For this review, take the finished solid that the model builds, in its own axes (mm). Face numbers are marked on the shaded views. A direction names the side the tool comes from. Coordinates: 2 decimals unless noted, no trailing zeros. Loops run counter-clockwise (first coordinate to the right, second up) from the corner with the lowest first, then second, coordinate; pieces in that order, holes last. Notation, with made-up numbers: (-38, 11) - (4, 11) arc R25 ccw to (4, 47) - close; hole circle Ø8 at (7, 44.5). An arc over 180 degrees is marked (long way). One line per item, written item: value. Start each with the question number.
1. To check wall thickness, follow line 1 (Z direction, x = 44.25, y = -91); line 2 (Z direction, x = 44, y = 46.5); line 3 (Z direction, x = 45.5, y = 78). State the ranges of each line that lie inside material, in increasing order. Write a range as from..to.
2. For the marked faces 1, 2 and 3, list the 3-axis set-ups (+Z, -Z, +X, -X, +Y, -Y) from which the entire face can be reached by the end or side of a thin tool; tool diameter is ignored.
3. The part is to be moulded in two halves that separate along Y. For the marked faces 4, 5 and 6, say which applies: released by +Y, released by -Y, zero draft, split by the parting line, or undercut.
4. Take a section at B-B, the plane z = -11. State the section outline as (x, y) points.
5. Take a section at C-C, the plane y = -70. State the section outline as (x, z) points, and give its area (3 significant figures).
6. Take a section at D-D, the plane x = 68. State the section outline as (y, z) points, and give its area (3 significant figures).
7. Insertion check: pin 1 (25 mm diameter, centred on x = 58.5, y = -33.5, fed in from +Z); pin 2 (1.8 mm diameter, centred on y = 0, z = 89.5, fed in from -X). Each pin has a flat end and moves straight along its axis. Give the tip position at first contact, or say it passes through.
8. Take a section at A-A, the plane x = 9.25. State the section outline as (y, z) points, and give its area (3 significant figures).
```python
from build123d import *

# Parameters (mm, degrees)
F1_DEPTH = 88.5
F2_R     = 3.4
F3_DEPTH = 30
F5_DEPTH = 208


with BuildPart() as f1:
    # F0 (on Right) → F1 (new body)
    with BuildSketch(Plane.YZ):
        Polygon((-74.5, 0), (68.5, 0), (56.952995, -20), (103.5, -20), (103.5, 85), (-104.5, 85), (-104.5, -20), (-74.5, -20), align=None)
    extrude(amount=F1_DEPTH)

    # F2 (on face) → F3 (cut, through all)
    with BuildSketch(Plane.XZ.offset(104.5)):
        with Locations((9.25, -11)):
            Circle(F2_R)
        with Locations((44.25, -11)):
            Circle(F2_R)
        with Locations((79.25, -11)):
            Circle(F2_R)
    extrude(amount=-F3_DEPTH, mode=Mode.SUBTRACT)

    # F4 (on face) → F5 (join, through all)
    with BuildSketch(Plane.XZ.offset(104.5)):
        Polygon((25, 91), (25, 85), (38, 85), (30.5, 91), align=None)
    extrude(amount=-F5_DEPTH)


solid = f1.part
```
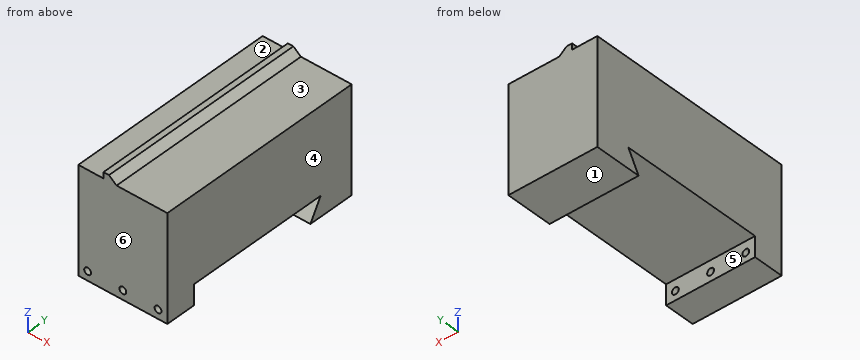
Solutions:
1. line 1: -20..-14.4, -7.6..85
1. line 2: 0..85
1. line 3: -20..85
2. face 1: -Z, +X, -X, +Y, -Y
2. face 2: +Z, -X, +Y, -Y
2. face 3: +Z, +X, +Y, -Y
3. face 4: zero draft
3. face 5: undercut
3. face 6: released by -Y
4. outline: (0, -104.5) - (5.85, -104.5) - (5.85, -74.5) - (0, -74.5) - close; (0, 62.15) - (88.5, 62.15) - (88.5, 103.5) - (0, 103.5) - close; (12.65, -104.5) - (40.85, -104.5) - (40.85, -74.5) - (12.65, -74.5) - close; (47.65, -104.5) - (75.85, -104.5) - (75.85, -74.5) - (47.65, -74.5) - close; (82.65, -104.5) - (88.5, -104.5) - (88.5, -74.5) - (82.65, -74.5) - close
5. outline: (0, 0) - (88.5, 0) - (88.5, 85) - (38, 85) - (30.5, 91) - (25, 91) - (25, 85) - (0, 85) - close
5. area: 7,580 mm2
6. outline: (-104.5, -20) - (-74.5, -20) - (-74.5, 0) - (68.5, 0) - (56.95, -20) - (103.5, -20) - (103.5, 85) - (-104.5, 85) - close
6. area: 19,100 mm2
7. pin 1: z = 85
7. pin 2: x = 25
8. outline: (-104.5, -20) - (-74.5, -20) - (-74.5, -14.4) - (-104.5, -14.4) - close; (-104.5, -7.6) - (-74.5, -7.6) - (-74.5, 0) - (68.5, 0) - (56.95, -20) - (103.5, -20) - (103.5, 85) - (-104.5, 85) - close
8. area: 18,900 mm2
